```python
from build123d import *

# Parameters (mm, degrees)
F1_DEPTH = 15
F2_R     = 3
F3_DEPTH = 8.001


with BuildPart() as f1:
    # F0 (on Front) → F1 (new body)
    with BuildSketch(Plane.XZ):
        Polygon((-4, 0), (0, 0), (4, 0), (7.5, 3.5), (7.5, 6), (4, 6), (4, 8), (0, 8), (-4, 8), (-4, 6), (-7.5, 6), (-7.5, 3.5), align=None)
    extrude(amount=F1_DEPTH)

    # F2 (on face) → F3 (cut, through all)
    with BuildSketch(Plane.XY.offset(8)):
        with Locations((0, -7.5)):
            Circle(F2_R)
    extrude(amount=-F3_DEPTH, mode=Mode.SUBTRACT)


solid = f1.part
```
The listing builds one solid part. Answer for the finished solid, in the listing's coordinates (mm). A direction names the side the tool comes from. Give positions to 0.01 mm unless a question says otherwise; leave off trailing zeros. Loops run counter-clockwise (first coordinate to the right, second up) from the corner with the lowest first, then second, coordinate; pieces in that order, holes last. Notation, with made-up numbers: M -38.5,0 L -32.5,0 A18 cw -32.5,28 Z; hole C 54.5,-3.5 d9. An arc over 180 degrees is marked long. One line per item, written item: value.
1. Section C-C on z = 1.25 is taken. Determine the outline of the cut face in (x, y).
Found:
outline: M -5.25,-15 L 5.25,-15 L 5.25,0 L -5.25,0 Z; hole C 0,-7.5 d6
2. Section D-D on y = -12.25 is taken. Determine the outline of the cut face in (x, z).
Found:
outline: M -7.5,3.5 L -4,0 L 4,0 L 7.5,3.5 L 7.5,6 L 4,6 L 4,8 L -4,8 L -4,6 L -7.5,6 Z
3. Section A-A on x = 0 is taken. Determine the outline of the cut face in (y, z), plus the area to 3 significant figures.
Found:
outline: M -15,0 L -10.5,0 L -10.5,8 L -15,8 Z; M -4.5,0 L 0,0 L 0,8 L -4.5,8 Z
area: 72.0 mm^2
4. For a pull along X with two mould halves and no side action, classify faces 1 (the face through (4, -7, 7)), 2 (the face through (-7.5, -7, 5)), 3 (the face through (-0.391, -4.526, 4.056)) as pulls with the +X half, pulls with the -X half, needs draft (parallel to the pull), parting line crosses it, or undercut.
Found:
face 1: pulls with the +X half
face 2: pulls with the -X half
face 3: undercut
5. Section B-B on y = -7.5 is taken. Determine the outline of the cut face in (x, z), plus the area to 4 significant figures.
Found:
outline: M -7.5,3.5 L -4,0 L -3,0 L -3,8 L -4,8 L -4,6 L -7.5,6 Z; M 3,0 L 4,0 L 7.5,3.5 L 7.5,6 L 4,6 L 4,8 L 3,8 Z
area: 45.75 mm^2
6. Find the intervals of material crossed by probe 1 along Y at (x, z) = (0, 4.75); probe 2 along X at (y, z) = (-13.25, 7); probe 3 along Y at (x, z) = (-2.5, 6), in increasing order.
Found:
probe 1: -15 to -10.5, -4.5 to 0
probe 2: -4 to 4
probe 3: -15 to -9.16, -5.84 to 0
7. For faces 4 (the face through (6, -7, 6)), 5 (the face through (7.5, -7, 5)), 6 (the face through (-4, -7, 7)), determine the directions among +Z, -Z, +X, -X, +Y, -Y from which every point of the face is accessible in a straight line to the end or side of a thin tool.
Found:
face 4: +Z, +X, +Y, -Y
face 5: +Z, -Z, +X, +Y, -Y
face 6: +Z, -X, +Y, -Y
8. Each of these flat-tipped pins is pushed along its axis until it touches: P1, Ø1.8, axis at x = -6.5, y = -9, coming from the +Z side; P2, Ø1.6, axis at y = -10.5, z = 7.5, coming from the -X side. Where does it stop, or does it pass through?
Found:
P1: z = 6
P2: x = -4
